```python
from build123d import *

# Parameters (mm, degrees)
SKETCH056_W     = 30
SKETCH056_H     = 32
SKETCH056_R     = 1.7
PAD037_DEPTH    = 10
SKETCH057_R     = 3.5
POCKET020_DEPTH = 5
POCKET020_TAPER = 20
SKETCH059_R     = 4.925
POCKET022_DEPTH = 32
SKETCH060_W     = 32
SKETCH060_H     = 10
PAD038_DEPTH    = 12
SKETCH062_R     = 1.575
POCKET024_DEPTH = 8
SKETCH086_R     = 3.975
POCKET037_DEPTH = 7


with BuildPart() as part:
    # Sketch056 → Pad037 (new body)
    with BuildSketch(Plane.XZ):
        Rectangle(SKETCH056_W, SKETCH056_H)
        with Locations((10, 4)):
            Circle(SKETCH056_R, mode=Mode.SUBTRACT)
        with Locations((10, -4)):
            Circle(SKETCH056_R, mode=Mode.SUBTRACT)
        with Locations((-10, 0)):
            Circle(SKETCH056_R, mode=Mode.SUBTRACT)
    extrude(amount=PAD037_DEPTH)

    # Sketch057 (on Face8 of Pad037) → Pocket020 (cut)
    with BuildSketch(Plane(origin=(0, 0, 0), x_dir=(1, 0, 0), z_dir=(0, 1, 0))):
        with Locations((-10, 0)):
            Circle(SKETCH057_R)
        with Locations((10, 4)):
            Circle(SKETCH057_R)
        with Locations((10, -4)):
            Circle(SKETCH057_R)
    extrude(amount=-POCKET020_DEPTH, taper=POCKET020_TAPER, mode=Mode.SUBTRACT)

    # Sketch059 (on Face1 of Pocket020) → Pocket022 (cut)
    with BuildSketch(Plane(origin=(0, 0, -16), x_dir=(1, 0, 0), z_dir=(0, 0, -1))):
        with Locations((0, 10)):
            Circle(SKETCH059_R)
    extrude(amount=-POCKET022_DEPTH, mode=Mode.SUBTRACT)

    # Sketch060 (on Face3 of Pocket022) → Pad038 (join)
    with BuildSketch(Plane(origin=(15, 0, 0), x_dir=(0, 0, 1), z_dir=(1, 0, 0))):
        with Locations((0, 5)):
            Rectangle(SKETCH060_W, SKETCH060_H)
    pad038 = extrude(amount=PAD038_DEPTH)

    # Sketch062 → Pocket024 (cut)
    with BuildSketch(Plane.XZ.offset(10)):
        with Locations((-10, 10)):
            Circle(SKETCH062_R)
        with Locations((-10, -10)):
            Circle(SKETCH062_R)
        with Locations((10, 10)):
            Circle(SKETCH062_R)
        with Locations((10, -10)):
            Circle(SKETCH062_R)
    extrude(amount=-POCKET024_DEPTH, mode=Mode.SUBTRACT)

    # Mirrored005: Pad038 across YZ
    add(pad038.mirror(Plane.YZ))

    # Sketch086 (on Face4 of Mirrored005) → Pocket037 (cut)
    with BuildSketch(Plane.XZ.offset(10)):
        with Locations((21, 0)):
            Circle(SKETCH086_R)
        with Locations((-21, 7)):
            Circle(SKETCH086_R)
        with Locations((-21, -7)):
            Circle(SKETCH086_R)
    extrude(amount=-POCKET037_DEPTH, mode=Mode.SUBTRACT)


with BuildPart() as part_1:
    # Body010 placement: moved
    add(part.part.moved(Location((-1, -43.5, 39.5))))


solid = part_1.part
```
Input: part model. Units: mm. Frame: model coordinates. A direction names the side the tool comes from. Give positions to 0.01 mm unless a question says otherwise; leave off trailing zeros. Order: outer loops, then holes, each group sorted by start corner. A loop starts at its lowest first (then second) coordinate and runs counter-clockwise, first axis right, second up.
1. Cut plane A-A (x = 9). Return loops of the section in (y, z) (3 decimals).
Computed:
outline: (-53.5, 23.5) - (-43.5, 23.5) - (-43.5, 32) - (-48.445, 33.8) - (-53.5, 33.8) - (-53.5, 31.075) - (-45.5, 31.075) - (-45.5, 27.925) - (-53.5, 27.925) - close; (-53.5, 37.2) - (-48.445, 37.2) - (-43.5, 39) - (-43.5, 40) - (-48.445, 41.8) - (-53.5, 41.8) - close; (-53.5, 45.2) - (-48.445, 45.2) - (-43.5, 47) - (-43.5, 55.5) - (-53.5, 55.5) - (-53.5, 51.075) - (-45.5, 51.075) - (-45.5, 47.925) - (-53.5, 47.925) - close
2. Set-up query: faces 1 (the face through (-1, -43.5, 39)), 2 (the face through (-22, -46.5, 47)). Return all of +Z, -Z, +X, -X, +Y, -Y with unobstructed straight access to the full face (end or side cutting, diameter ignored); none if empty.
Computed:
face 1: +Z, -Z, +X, -X, +Y
face 2: -Y
3. Cut plane D-D (z = 49.5). Return loops of the section in (x, y) (3 decimals), and give its area (3 significant figures).
Computed:
outline: (-28, -53.5) - (-24.608, -53.5) - (-24.608, -46.5) - (-19.392, -46.5) - (-19.392, -53.5) - (-12.575, -53.5) - (-12.575, -45.5) - (-9.425, -45.5) - (-9.425, -53.5) - (-5.925, -53.5) arc R4.925 cw to (3.925, -53.5) - (7.425, -53.5) - (7.425, -45.5) - (10.575, -45.5) - (10.575, -53.5) - (26, -53.5) - (26, -43.5) - (-28, -43.5) - close
area: 415 mm2
4. Pin query (flat end, axial travel): pin 1 Ø2 at (x, z) = (-11, 39.5) entering from +Y; pin 2 Ø0.9 at (x, z) = (9.5, 49.5) entering from -Y; pin 3 Ø2.5 at (x, z) = (21.5, 40.5) entering from -Y. Return the tip coordinate at first contact, or that it passes through.
Computed:
pin 1: passes through
pin 2: stops at y = -45.5
pin 3: stops at y = -46.5
5. Cut plane B-B (y = -51.75). State how many separate pieces and enclosed holes the cut face has, and give its area (3 significant figures).
Computed:
separate pieces: 2
enclosed holes: 10
area: 1,230 mm2
6. Line query: probe 1 along Z at (x, y) = (-22, -50.75) (3 decimals); probe 2 along Z at (x, y) = (-11, -49.5) (3 decimals); probe 3 along Z at (x, y) = (9, -52) (3 decimals). Output: solid intervals per line, ascending.
Computed:
probe 1: z = 23.5 to 28.525, 36.475 to 42.525, 50.475 to 55.5
probe 2: z = 23.5 to 27.925, 31.075 to 37.8, 41.2 to 47.925, 51.075 to 55.5
probe 3: z = 23.5 to 27.925, 31.075 to 33.8, 37.2 to 41.8, 45.2 to 47.925, 51.075 to 55.5
7. Draft query along Z for faces 3 (the face through (19.48, -50.05, 43.44)), 4 (the face through (-1, -48, 23.5)), 5 (the face through (-17, -53.5, 39)). Return one class per face: released by +Z, released by -Z, zero draft, split by the parting line, or undercut.
Computed:
face 3: undercut
face 4: released by -Z
face 5: zero draft
